```python
from build123d import *

# Parameters (mm, degrees)
BOSS_EXTRUDE1_DEPTH = 32.5
CUT_EXTRUDE1_DEPTH  = 31.122
SKETCH4_R           = 1.05
BOSS_EXTRUDE2_DEPTH = 1.5
SKETCH5_R           = 1.05
BOSS_EXTRUDE3_DEPTH = 2
FILLET1_R           = 1
SKETCH6_W           = 15
SKETCH6_H           = 2.5
BOSS_EXTRUDE4_DEPTH = 2


with BuildPart() as part:
    # Sketch2 → Boss-Extrude1 (new body)
    with BuildSketch(Plane(origin=(0, 0, 0), x_dir=(1, 0, 0), z_dir=(0, 1, 0))):
        Polygon((15.061, 0), (15.061, 32), (12.561, 32), (12.561, 2.5), (-12.561, 2.5), (-12.561, 32), (-15.061, 32), (-15.061, 0), align=None)
    extrude(amount=BOSS_EXTRUDE1_DEPTH)

    # Sketch3 → Cut-Extrude1 (cut, through all)
    with BuildSketch(Plane(origin=(15.061, 0, 0), x_dir=(0, 0, -1), z_dir=(1, 0, 0))):
        Polygon((32, 10), (12.5, 32.5), (32, 32.5), align=None)
    extrude(amount=-CUT_EXTRUDE1_DEPTH, mode=Mode.SUBTRACT)

    # Sketch4 → Boss-Extrude2 (add)
    with BuildSketch(Plane.XZ):
        Polygon((-15.061, 0), (-15.061, -32), (-10.061, -32), (-8.061, -29.4695), (-12.561, -25), (-12.561, -10), (-7.5, -6), (7.5, -6), (12.561, -10), (12.561, -25), (8.061, -29.4695), (10.061, -32), (15.061, -32), (15.061, 0), align=None)
        with Locations((-10.2499, -4.95)):
            Circle(SKETCH4_R, mode=Mode.SUBTRACT)
        with Locations((-10.2499, -29.4)):
            Circle(SKETCH4_R, mode=Mode.SUBTRACT)
        with Locations((10.2499, -29.4)):
            Circle(SKETCH4_R, mode=Mode.SUBTRACT)
        with Locations((10.2499, -4.95)):
            Circle(SKETCH4_R, mode=Mode.SUBTRACT)
    extrude(amount=BOSS_EXTRUDE2_DEPTH)

    # Sketch5 → Boss-Extrude3 (add)
    with BuildSketch(Plane(origin=(0, 32.5, 0), x_dir=(1, 0, 0), z_dir=(0, 1, 0))):
        Polygon((-15.061, 12), (-10.2499, 12), (-7.5, 10), (-7.5, 0), (-15.061, 0), align=None)
        with Locations((-10.2499, 8.7)):
            Circle(SKETCH5_R, mode=Mode.SUBTRACT)
        Polygon((15.061, 12), (10.2499, 12), (7.5, 10), (7.5, 0), (15.061, 0), align=None)
        with Locations((10.2499, 8.7)):
            Circle(SKETCH5_R, mode=Mode.SUBTRACT)
    extrude(amount=BOSS_EXTRUDE3_DEPTH)

    # Fillet1
    fillet1_edges = [part.edges().sort_by_distance(p)[0] for p in [
        (-8.061, -0.75, -29.4695),
        (8.061, -0.75, -29.4695),
    ]]
    fillet(fillet1_edges, radius=FILLET1_R)

    # Sketch6 → Boss-Extrude4 (add)
    with BuildSketch(Plane(origin=(0, 34.5, 0), x_dir=(1, 0, 0), z_dir=(0, 1, 0))):
        with Locations((0, 1.25)):
            Rectangle(SKETCH6_W, SKETCH6_H)
    extrude(amount=-BOSS_EXTRUDE4_DEPTH)


solid = part.part
```
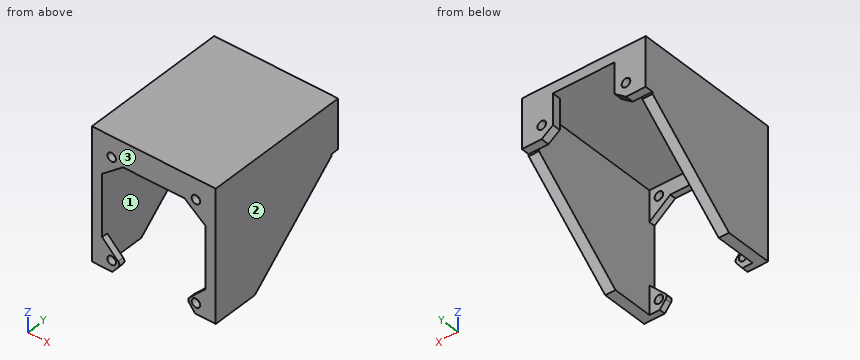
Geometry check sheet. Reference: the model listing, model coordinates, mm. Face numbers are marked on the shaded views. Coordinates: 2 decimals unless noted, no trailing zeros. Order: outer loops, then holes, each group sorted by start corner. A loop starts at its lowest first (then second) coordinate and runs counter-clockwise, first axis right, second up. Notation, with made-up numbers: (15, -7.75) - (41, -7.75) arc R15 ccw to (41, 6.25) - close; hole circle Ø7 at (-9.75, 71.5). An arc over 180 degrees is marked (long way). Answer as a JSON object with one key per item and string values. Group by question number.
Item 1: Depth check by flat-ended pin: pin 1 Ø2.5 at (x, z) = (10.25, -29.4) entering from +Y; pin 2 Ø1 at (y, z) = (20, -24.5) entering from +X; pin 3 Ø1.3 at (x, z) = (-10.25, -4.95) entering from -Y; pin 4 Ø0.6 at (x, z) = (-14, -12.5) entering from +Y. Enter the tip coordinate at first touch or a pass-through.
Item 2: Sectioned sample at A-A, the plane z = -4.95. Record the cut outline in (x, y).
Item 3: Sectioned sample at C-C, the plane y = 3. Record the cut outline in (x, z).
Item 4: Scan lines: probe 1 along X at (y, z) = (17.5, -21); probe 2 along X at (y, z) = (-1, -29); probe 3 along X at (y, z) = (-1, -4). Record each from-to range of solid material in increasing order.
Item 5: Sectioned sample at B-B, the plane z = -29.4. Record the cut outline in (x, y).
Item 6: Sectioned sample at D-D, the plane z = -21.5. Record the cut outline in (x, y).
Item 7: Draft check along Y on the marked faces 1, 2 and 3. Enter one of: +Y half, -Y half, draft (parallel to the pull), parting line (faces both ways), or undercut.
Resolved:
{
 "1": {"pin 1": "y = 0", "pin 2": "through", "pin 3": "y = 32.5", "pin 4": "y = 32.5"},
 "2": {"outline": "(-15.06, -1.5) - (-11.3, -1.5) - (-11.3, 0) - (-12.56, 0) - (-12.56, 32.5) - (-7.5, 32.5) - (-7.5, 34.5) - (-15.06, 34.5) - close; (-9.2, -1.5) - (9.2, -1.5) - (9.2, 0) - (-9.2, 0) - close; (7.5, 32.5) - (12.56, 32.5) - (12.56, 0) - (11.3, 0) - (11.3, -1.5) - (15.06, -1.5) - (15.06, 34.5) - (7.5, 34.5) - close"},
 "3": {"outline": "(-15.06, -32) - (-12.56, -32) - (-12.56, -2.5) - (12.56, -2.5) - (12.56, -32) - (15.06, -32) - (15.06, 0) - (-15.06, 0) - close"},
 "4": {"probe 1": "-15.06 to -12.56, 12.56 to 15.06", "probe 2": "-15.06 to -11.22, -9.28 to -8.56, 8.56 to 9.28, 11.22 to 15.06", "probe 3": "-15.06 to -10.7, -9.8 to 9.8, 10.7 to 15.06"},
 "5": {"outline": "(-15.06, -1.5) - (-11.3, -1.5) - (-11.3, 0) - (-12.56, 0) - (-12.56, 13) - (-15.06, 13) - close; (-9.2, -1.5) - (-8.41, -1.5) - (-8.41, 0) - (-9.2, 0) - close; (8.41, -1.5) - (9.2, -1.5) - (9.2, 0) - (8.41, 0) - close; (11.3, -1.5) - (15.06, -1.5) - (15.06, 13) - (12.56, 13) - (12.56, 0) - (11.3, 0) - close"},
 "6": {"outline": "(-15.06, -1.5) - (-12.56, -1.5) - (-12.56, 22.12) - (-15.06, 22.12) - close; (12.56, -1.5) - (15.06, -1.5) - (15.06, 22.12) - (12.56, 22.12) - close"},
 "7": {"face 1": "undercut", "face 2": "draft", "face 3": "-Y half"}
}
